Read the model definition and answer for the solid it produces. Units are mm, in the model's axes. A direction names the side the tool comes from. Round coordinates to 2 decimals unless told otherwise and drop trailing zeros. Write each loop counter-clockwise with the first axis right and the second up, starting at its lowest first coordinate (ties: lowest second). Pieces come first, ordered by that corner, then holes.
from build123d import *

# Parameters (mm, degrees)
F0_W     = 76.2
F0_H     = 50.8
F1_DEPTH = 12.7
F2_W     = 12.7
F2_H     = 25.4
F3_DEPTH = 76.2
F5_DEPTH = 12.7
F7_DEPTH = 30.48


with BuildPart() as f1:
    # F0 (on Top) → F1 (new body)
    with BuildSketch(Plane.XY):
        with Locations((-38.1, 25.4)):
            Rectangle(F0_W, F0_H)
    extrude(amount=F1_DEPTH)

    # F2 (on face) → F3 (join)
    with BuildSketch(Plane.YZ):
        with Locations((44.45, 25.4)):
            Rectangle(F2_W, F2_H)
    extrude(amount=-F3_DEPTH)

    # F4 (on face) → F5 (join)
    with BuildSketch(Plane.XZ.offset(-38.1)):
        with BuildLine():
            Line((-19.05, 38.1), (0, 38.1))
            ThreePointArc((0, 38.1), (-38.1, 76.2), (-76.2, 38.1))
            Line((-76.2, 38.1), (-57.15, 38.1))
            ThreePointArc((-57.15, 38.1), (-38.1, 57.15), (-19.05, 38.1))
        make_face()
    extrude(amount=-F5_DEPTH)

    # F6 (on face) → F7 (cut)
    with BuildSketch(Plane.XZ.offset(-38.1)):
        with BuildLine():
            Line((-57.15, 38.1), (-19.05, 38.1))
            ThreePointArc((-19.05, 38.1), (-38.1, 57.15), (-57.15, 38.1))
        make_face()
        with BuildLine():
            ThreePointArc((-57.15, 38.1), (-38.1, 19.05), (-19.05, 38.1))
            Line((-19.05, 38.1), (-57.15, 38.1))
        make_face()
    extrude(amount=-F7_DEPTH, mode=Mode.SUBTRACT)


solid = f1.part
Q1. Determine the mould class of faces 1 (the flat face through (-76.2, 31, 11)), 2 (the flat face through (-39, 19, 12.7)), 3 (the flat face through (0, 31, 11)), 4 (the cylindrical face through (-35.62, 44.361, 19.212)) for opening direction X: pulls with the +X half, pulls with the -X half, needs draft (parallel to the pull), parting line crosses it, or undercut.
Verdict:
face 1: pulls with the -X half
face 2: needs draft
face 3: pulls with the +X half
face 4: undercut
Q2. Section B-B (z = 21) is taken. Determine the outline of the cut face in (x, y).
Verdict:
outline: (-76.2, 38.1) - (-46.5, 38.1) - (-46.5, 50.8) - (-76.2, 50.8) - close; (-29.7, 38.1) - (0, 38.1) - (0, 50.8) - (-29.7, 50.8) - close
Q3. Straight lines are drawn through the part: probe 1 along X at (y, z) = (41.75, 38.1); probe 2 along Z at (x, y) = (-38, 42); probe 3 along Y at (x, z) = (-54, 21). For each, find the intervals that lie inside material, in ascending order.
Verdict:
probe 1: x = -76.2 to -57.15, -19.05 to 0
probe 2: z = 0 to 19.05, 57.15 to 76.2
probe 3: y = 38.1 to 50.8
Q4. Section D-D (x = -27) is taken. Determine the outline of the cut face in (y, z).
Verdict:
outline: (0, 0) - (50.8, 0) - (50.8, 22.62) - (38.1, 22.62) - (38.1, 12.7) - (0, 12.7) - close; (38.1, 53.58) - (50.8, 53.58) - (50.8, 74.55) - (38.1, 74.55) - close
Q5. Flat-ended cylindrical pins translate along their axes: pin 1 Ø4 at (x, z) = (-21, 56.5) entering from -Y; pin 2 Ø1.5 at (x, y) = (-56.5, 32) entering from +Z. Find the tip coordinate at first contact, or state that the pin passes through.
Verdict:
pin 1: stops at y = 38.1
pin 2: stops at z = 12.7
Q6. Which of the six approach directions +Z, -Z, +X, -X, +Y, -Y give full straight-line access (tool end or side, diameter ignored) to faces 5 (the cylindrical face through (-37.26, 44.36, 76.19)), 6 (the flat face through (-39, 38.1, 59))?
Verdict:
face 5: +Z, +Y, -Y
face 6: +Z, +X, -X, -Y
Q7. Section A-A (x = -38.1) is taken. Determine the outline of the cut face in (y, z).
Verdict:
outline: (0, 0) - (50.8, 0) - (50.8, 19.05) - (38.1, 19.05) - (38.1, 12.7) - (0, 12.7) - close; (38.1, 57.15) - (50.8, 57.15) - (50.8, 76.2) - (38.1, 76.2) - close
Q8. Section C-C (y = 6.5) is taken. Determine the outline of the cut face in (x, z), then the cut area to 3 significant figures.
Verdict:
outline: (-76.2, 0) - (0, 0) - (0, 12.7) - (-76.2, 12.7) - close
area: 968 mm2
